Read the model definition and answer for the solid it produces. Units are mm, in the model's axes. Give positions to 0.01 mm unless a question says otherwise; leave off trailing zeros. Order: outer loops, then holes, each group sorted by start corner. A loop starts at its lowest first (then second) coordinate and runs counter-clockwise, first axis right, second up. Notation, with made-up numbers: (56.5, 47.25) - (83.5, 47.25) arc R17 cw to (83.5, 74.25) - close; hole circle Ø4 at (-4.5, -23). An arc over 180 degrees is marked (long way). Answer as CSV lines item,"result". Start each with the question number.
from build123d import *

# Parameters (mm, degrees)
F0_W     = 60
F0_H     = 20
F1_DEPTH = 4
F2_D     = 10.2
F3_R     = 5


with BuildPart() as f1:
    # F0 (on Top) → F1 (new body)
    with BuildSketch(Plane.XY):
        Rectangle(F0_W, F0_H)
    extrude(amount=F1_DEPTH)

    # F2 (through all)
    with Locations(Plane(origin=(0, 0, 0), x_dir=(1, 0, 0), z_dir=(0, 0, -1))):
        with Locations((-20, 0), (20, 0)):
            Hole(F2_D / 2)

    # F3
    f3_edges = [f1.edges().sort_by_distance(p)[0] for p in [
        (-30, 10, 2),
        (-30, -10, 2),
        (30, 10, 2),
        (30, -10, 2),
    ]]
    fillet(f3_edges, radius=F3_R)


solid = f1.part
(1) Section C-C, the plane y = -2.5 is taken. Write down the section's boundary in (x, z), and give its area (3 significant figures).
(2) Straight lines are drawn through the part: line 1 (Y direction, x = -20, z = 2.45); line 2 (X direction, y = -3.5, z = 1.5); line 3 (X direction, y = -4, z = 2.05). For each, find the intervals that lie inside material, in ascending order. Write a range as [from, to].
(3) Determine the mould class of faces 1 (the cylindrical face through (-29, -8, 2)), 2 (the cylindrical face through (24.05, 3.1, 2.03)), 3 (the cylindrical face through (-29, 8, 2)), 4 (the cylindrical face through (-24.864, -1.532, 2.028)) for opening direction Y: released by +Y, released by -Y, zero draft, split by the parting line, or undercut.
(4) Section B-B, the plane z = 0.85 is taken. Write down the section's boundary in (x, y), and give its area (3 significant figures).
(5) Section A-A, the plane x = -20 is taken. Write down the section's boundary in (y, z), and give its area (3 significant figures).
(6) Section D-D, the plane x = 23 is taken. Write down the section's boundary in (y, z).
Checks:
1,outline,"(-30, 0) - (-24.45, 0) - (-24.45, 4) - (-30, 4) - close; (-15.55, 0) - (15.55, 0) - (15.55, 4) - (-15.55, 4) - close; (24.45, 0) - (30, 0) - (30, 4) - (24.45, 4) - close"
1,area,"169 mm²"
2,line 1,"y = [-10, -5.1], [5.1, 10]"
2,line 2,"x = [-30, -23.71], [-16.29, 16.29], [23.71, 30]"
2,line 3,"x = [-30, -23.16], [-16.84, 16.84], [23.16, 30]"
3,face 1,"released by -Y"
3,face 2,"undercut"
3,face 3,"released by +Y"
3,face 4,"undercut"
4,outline,"(-30, -5) arc R5 ccw to (-25, -10) - (25, -10) arc R5 ccw to (30, -5) - (30, 5) arc R5 ccw to (25, 10) - (-25, 10) arc R5 ccw to (-30, 5) - close; hole circle Ø10.2 at (-20, 0); hole circle Ø10.2 at (20, 0)"
4,area,"1,020 mm²"
5,outline,"(-10, 0) - (-5.1, 0) - (-5.1, 4) - (-10, 4) - close; (5.1, 0) - (10, 0) - (10, 4) - (5.1, 4) - close"
5,area,"39.2 mm²"
6,outline,"(-10, 0) - (-4.12, 0) - (-4.12, 4) - (-10, 4) - close; (4.12, 0) - (10, 0) - (10, 4) - (4.12, 4) - close"
